Geometry: see drawing. Coordinates: mm, zero at the bounding-box minimum. Round coordinates to 2 decimals unless told otherwise and drop trailing zeros. Order: outer loops, then holes, each group sorted by start corner. A loop starts at its lowest first (then second) coordinate and runs counter-clockwise, first axis right, second up. Notation, with made-up numbers: M -19.5,41 L 8.5,41 A28 cw 8.5,62 Z; hole C 35,0.25 d11. An arc over 180 degrees is marked long. Answer in a Markdown table with one row per item. Add a question column.
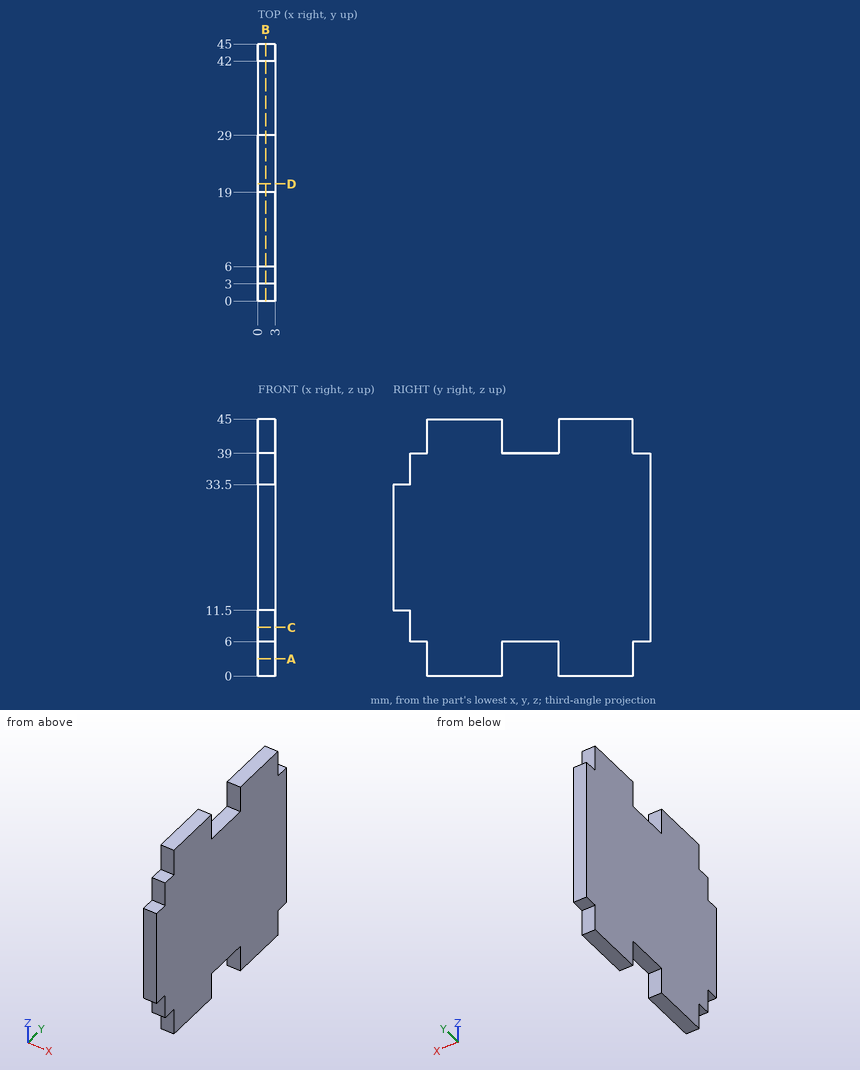
(1) Cut plane A-A (z = 3). Return loops of the section in (x, y).
(2) Line query: line 1 (Y direction, x = 2.6, z = 4.5); line 2 (Z direction, x = 2.45, y = 2); line 3 (Y direction, x = 1, z = 10.5). Output: solid intervals per line, ascending. Write a range as from..to.
(3) Cut plane D-D (y = 20.5). Return loops of the section in (x, z), and give its area (3 significant figures).
(4) Cut plane C-C (z = 8.5). Return loops of the section in (x, y).
(5) Pin query (flat end, axial travel): pin 1 (0.9 mm diameter, centred on x = 2, z = 42, fed in from +Y); pin 2 (1.5 mm diameter, centred on y = 40, z = 40, fed in from -X); pin 3 (0.9 mm diameter, centred on x = 2, y = 5, fed in from -Z); pin 4 (1.5 mm diameter, centred on x = 2, z = 3.5, fed in from -Y). Return the tip coordinate at first contact, or that it passes through.
(6) Cut plane B-B (x = 1.35). Return loops of the section in (y, z).
Answer list:
| question | item | result |
|---|---|---|
| 1 | outline | M 0,6 L 3,6 L 3,19 L 0,19 Z; M 0,29 L 3,29 L 3,42 L 0,42 Z |
| 2 | line 1 | 6..19, 29..42 |
| 2 | line 2 | 11.5..33.5 |
| 2 | line 3 | 3..45 |
| 3 | outline | M 0,6 L 3,6 L 3,39 L 0,39 Z |
| 3 | area | 99.0 mm² |
| 4 | outline | M 0,3 L 3,3 L 3,45 L 0,45 Z |
| 5 | pin 1 | y = 42 |
| 5 | pin 2 | x = 0 |
| 5 | pin 3 | z = 6 |
| 5 | pin 4 | y = 6 |
| 6 | outline | M 0,11.5 L 3,11.5 L 3,6 L 6,6 L 6,0 L 19,0 L 19,6 L 29,6 L 29,0 L 42,0 L 42,6 L 45,6 L 45,39 L 42,39 L 42,45 L 29,45 L 29,39 L 19,39 L 19,45 L 6,45 L 6,39 L 3,39 L 3,33.5 L 0,33.5 Z |
